```python
from build123d import *

# Parameters (mm, degrees)
F0_R     = 19.3675985609
F1_DEPTH = 9.9377613515
F2_W     = 53.0373156071
F2_H     = 49.859970808
F3_DEPTH = 8.5315406322
F5_D     = 25.4
F6_DEPTH = 27.8559215367
F7_SIZE  = 5.08
F8_SIZE  = 5.08


with BuildPart() as f1:
    # F0 (on Top) → F1 (new body)
    with BuildSketch(Plane.XY):
        Circle(F0_R)
    extrude(amount=F1_DEPTH)

    # F2 (on Top) → F3 (join)
    with BuildSketch(Plane.XY):
        Rectangle(F2_W, F2_H)
    extrude(amount=-F3_DEPTH)

    # F5 (through all)
    with Locations(Plane(origin=(0, 0, -8.5315406322), x_dir=(1, 0, 0), z_dir=(0, 0, -1))):
        with Locations((0, 0)):
            Hole(F5_D / 2)

    # F6 (add): a face of the model
    f6_faces = [f1.faces().sort_by_distance(p)[0] for p in [
        (-18.8198001498, 0, 9.9377613515),
    ]]
    extrude(f6_faces, amount=F6_DEPTH)

    # F7
    f7_edges = [f1.edges().sort_by_distance(p)[0] for p in [
        (-19.367599, 0, 37.793683),
    ]]
    chamfer(f7_edges, length=F7_SIZE)

    # F8
    f8_edges = [f1.edges().sort_by_distance(p)[0] for p in [
        (26.518658, 0, 0),
        (0, -24.929985, 0),
        (-26.518658, 0, 0),
        (0, 24.929985, 0),
    ]]
    chamfer(f8_edges, length=F8_SIZE)


solid = f1.part
```
Check sheet for the modelled part. Datum: model origin and axes. Units: mm. A direction names the side the tool comes from. Round coordinates to 2 decimals unless told otherwise and drop trailing zeros. Order: outer loops, then holes, each group sorted by start corner. A loop starts at its lowest first (then second) coordinate and runs counter-clockwise, first axis right, second up.
1) Scan lines: line 1 (Y direction, x = 0, z = 1); line 2 (Z direction, x = -19, y = 19); line 3 (X direction, y = -5.5, z = 30). Record each from-to range of solid material in increasing order.
2) Go/stop test with flat-tipped pins: pin 1 Ø1.5 at (x, y) = (2.5, -19.5) entering from +Z; pin 2 Ø5 at (x, z) = (-13, 26) entering from +Y; pin 3 Ø2 at (x, z) = (4.5, 26.5) entering from +Y. Record where each tip stops, or that it passes through.
3) Tool access check on faces 1 (the flat face through (-14.4, 13.3, 0)), 2 (the flat face through (-0.37, -22.43, -2.58)). Record the directions out of +Z, -Z, +X, -X, +Y, -Y that give a thin tool (end or side, any length) a straight path to the whole face; none if there is none.
4) Section check D-D (x = -20.5). Record the boundary of the cut face in (y, z), and give its area (3 significant figures).
5) Section check C-C (z = 30). Record the boundary of the cut face in (x, y), and give its area (3 significant figures).
6) Section check B-B (y = 0). Record the boundary of the cut face in (x, z).
7) Section check A-A (x = 0). Record the boundary of the cut face in (y, z), and give its area (3 significant figures).
Result:
1. line 1: y = -19.37 to -12.7, 12.7 to 19.37
1. line 2: z = -8.53 to 0
1. line 3: x = -18.57 to -11.45, 11.45 to 18.57
2. pin 1: stops at z = 33.17
2. pin 2: stops at y = 16.27
2. pin 3: stops at y = 19.05
3. face 1: +Z
3. face 2: +Z, +X, -X, -Y
4. outline: (-24.93, -8.53) - (24.93, -8.53) - (24.93, -5.08) - (19.85, 0) - (-19.85, 0) - (-24.93, -5.08) - close
4. area: 400 mm2
5. outline: circle Ø38.74 at (0, 0); hole circle Ø25.4 at (0, 0)
5. area: 672 mm2
6. outline: (-26.52, -8.53) - (-12.7, -8.53) - (-12.7, 37.79) - (-14.29, 37.79) - (-19.37, 32.71) - (-19.37, 0) - (-21.44, 0) - (-26.52, -5.08) - close; (12.7, -8.53) - (26.52, -8.53) - (26.52, -5.08) - (21.44, 0) - (19.37, 0) - (19.37, 32.71) - (14.29, 37.79) - (12.7, 37.79) - close
7. outline: (-24.93, -8.53) - (-12.7, -8.53) - (-12.7, 37.79) - (-14.29, 37.79) - (-19.37, 32.71) - (-19.37, 0) - (-19.85, 0) - (-24.93, -5.08) - close; (12.7, -8.53) - (24.93, -8.53) - (24.93, -5.08) - (19.85, 0) - (19.37, 0) - (19.37, 32.71) - (14.29, 37.79) - (12.7, 37.79) - close
7. area: 661 mm2
